The model under review builds one solid part; all positions refer to its coordinate system, in mm. A direction names the side the tool comes from. Give positions to 0.01 mm unless a question says otherwise; leave off trailing zeros. Order: outer loops, then holes, each group sorted by start corner. A loop starts at its lowest first (then second) coordinate and runs counter-clockwise, first axis right, second up. Notation, with made-up numbers: (59, -39) - (86, -39) arc R26 cw to (86, -20) - close; hole circle Ø1 at (74, 89.25). An arc over 180 degrees is marked (long way). Use CSV: the item, a comma, the result in double quotes. Start each with the question number.
1. For pin 1 (2.5 mm diameter, centred on x = -5.5, z = 7, fed in from +Y); pin 2 (5 mm diameter, centred on x = -13, z = 1, fed in from +Y); pin 3 (4.5 mm diameter, centred on x = 11.5, y = -73, fed in from +Z), all flat-tipped, find the tip position at first contact; note any pin that passes through.
2. To check wall thickness, follow line 1 (X direction, y = -77, z = 5.75); line 2 (Y direction, x = 16, z = 9.5); line 3 (Y direction, x = -3, z = 7.5). State the ranges of each line that lie inside material, in increasing order. Write a range as [from, to].
3. Machinability: for faces 1 (the flat face through (-3.26, -37.7, 5.01)), 2 (the flat face through (6, -73, 7.62)), 3 (the flat face through (6, -83, 0)), which of the approach directions +Z, -Z, +X, -X, +Y, -Y give a long, thin tool a straight path to every point of the face, cutting with its end or side? Answer none if there is none.
4. Take a section at C-C, the plane y = -70. State the section outline as (x, z) points.
5. Take a section at B-B, the plane x = 3.5. State the section outline as (y, z) points, then the cut area to 3 significant figures.
6. Draft analysis for pull direction Y (two halves, no side actions). For faces 4 (the flat face through (6, -100, 10.16)), 5 (the flat face through (6.62, -39.04, 5.01)), 6 (the flat face through (-8.671, -75, 4)), 7 (the flat face through (-7.796, -38.047, 5.009)), state which applies: released by +Y, released by -Y, zero draft, split by the parting line, or undercut.
7. Take a section at A-A, the plane z = 4. State the section outline as (x, y) points, then the cut area to 3 significant figures.
```python
from build123d import *

# Parameters (mm, degrees)
F1_DEPTH = 10.16
F2_DEPTH = 7.62
F0_W     = 7.62
F0_H     = 5.08
F3_DEPTH = 10.16


with BuildPart() as f1:
    # F0 (on Top) → F1 (new body)
    with BuildSketch(Plane.XY):
        Polygon((35.535632, -55.732704), (-23.123154, -21.866039), (-23.123154, -68.221039), (35.535632, -68.221039), align=None)
        Polygon((-11.14219, -36.1156), (-8.60219, -31.716191), (-2.003076, -35.526191), (-4.543076, -39.9256), align=None, mode=Mode.SUBTRACT)
        Polygon((17.212002, -52.4859), (10.612888, -48.6759), (13.152888, -44.276491), (19.752002, -48.086491), align=None, mode=Mode.SUBTRACT)
    extrude(amount=F1_DEPTH)

    # F0 (on Top) → F2 (join)
    with BuildSketch(Plane.XY):
        Polygon((35.535632, -68.221039), (-23.123154, -68.221039), (-23.123154, -77.111039), (-8.670554, -77.111039), (-8.670554, -72.031039), (-1.050554, -72.031039), (-1.050554, -77.111039), (13.402046, -77.111039), (13.402046, -72.031039), (21.022046, -72.031039), (21.022046, -77.111039), (35.535632, -77.111039), align=None)
    extrude(amount=F2_DEPTH)

    # F0 (on Top) → F3 (join)
    with BuildSketch(Plane.XY):
        Polygon((-8.670554, -77.111039), (-23.123154, -77.111039), (-23.123154, -123.466039), (8.804092, -123.466039), (25.314092, -123.466039), (35.535632, -123.466039), (35.535632, -77.111039), (21.022046, -77.111039), (13.402046, -77.111039), (-1.050554, -77.111039), align=None)
        with Locations((-4.860554, -120.291039)):
            Rectangle(F0_W, F0_H, mode=Mode.SUBTRACT)
        with Locations((17.212046, -120.304264)):
            Rectangle(F0_W, F0_H, mode=Mode.SUBTRACT)
    extrude(amount=F3_DEPTH)


solid = f1.part
```
Determined:
1,pin 1,"stops at y = -31.32"
1,pin 2,"stops at y = -26.27"
1,pin 3,"stops at z = 7.62"
2,line 1,"x = [-23.12, -8.67], [-1.05, 13.4], [21.02, 35.54]"
2,line 2,"y = [-123.47, -122.84], [-117.76, -77.11], [-68.22, -51.79], [-45.92, -44.45]"
2,line 3,"y = [-123.47, -122.83], [-117.75, -77.11], [-72.03, -37.25], [-34.95, -33.48]"
3,face 1,"+Z, -Z"
3,face 2,"+Z, +X, -X"
3,face 3,"-Z, +X, -X, +Y, -Y"
4,outline,"(-23.12, 0) - (35.54, 0) - (35.54, 7.62) - (-23.12, 7.62) - close"
5,outline,"(-123.47, 0) - (-37.24, 0) - (-37.24, 10.16) - (-68.22, 10.16) - (-68.22, 7.62) - (-77.11, 7.62) - (-77.11, 10.16) - (-123.47, 10.16) - close"
5,area,"854 mm²"
6,face 4,"zero draft"
6,face 5,"released by +Y"
6,face 6,"undercut"
6,face 7,"undercut"
7,outline,"(-23.12, -123.47) - (35.54, -123.47) - (35.54, -55.73) - (-23.12, -21.87) - close; hole (-11.14, -36.12) - (-4.54, -39.93) - (-2, -35.53) - (-8.6, -31.72) - close; hole (-8.67, -122.83) - (-1.05, -122.83) - (-1.05, -117.75) - (-8.67, -117.75) - close; hole (-8.67, -77.11) - (-1.05, -77.11) - (-1.05, -72.03) - (-8.67, -72.03) - close; hole (10.61, -48.68) - (17.21, -52.49) - (19.75, -48.09) - (13.15, -44.28) - close; hole (13.4, -122.84) - (21.02, -122.84) - (21.02, -117.76) - (13.4, -117.76) - close; hole (13.4, -77.11) - (21.02, -77.11) - (21.02, -72.03) - (13.4, -72.03) - close"
7,area,"4,730 mm²"
